from build123d import *

# Parameters (mm, degrees)
BOSS_EXTRUDE1_DEPTH = 8
HOLE1_D             = 3.2
HOLE1_CSINK_D       = 6
HOLE1_CSINK_ANGLE   = 90
FILLET1_R           = 5


with BuildPart() as part:
    # Sketch1 → Boss-Extrude1 (new body)
    with BuildSketch(Plane.XY):
        with BuildLine():
            Line((-13.754245124, 7.360756827), (-35.078110692, 7.360756827))
            Line((-35.078110692, 7.360756827), (-35.078110692, 1.360756827))
            Line((-35.078110692, 1.360756827), (-25.078110692, 1.360756827))
            Line((-25.078110692, 1.360756827), (-25.078110692, 4.360756827))
            Line((-25.078110692, 4.360756827), (-11.981080915, 4.360756827))
            ThreePointArc((-11.981080915, 4.360756827), (0, 12.75), (11.981080915, 4.360756827))
            Line((11.981080915, 4.360756827), (25.078110692, 4.360756827))
            Line((25.078110692, 4.360756827), (25.078110692, 1.360756827))
            Line((25.078110692, 1.360756827), (35.078110692, 1.360756827))
            Line((35.078110692, 1.360756827), (35.078110692, 7.360756827))
            Line((35.078110692, 7.360756827), (13.754245124, 7.360756827))
            ThreePointArc((13.754245124, 7.360756827), (0, 15.6), (-13.754245124, 7.360756827))
        make_face()
    extrude(amount=BOSS_EXTRUDE1_DEPTH)

    # Hole1 (through all)
    with Locations(Plane(origin=(-21.078110692, 7.360756827, 4), x_dir=(1, 0, 0), z_dir=(0, 1, 0))):
        with Locations((0, 0), (42.156221384, 0), (-10, 0), (52.156221384, 0)):
            CounterSinkHole(HOLE1_D / 2, HOLE1_CSINK_D / 2, counter_sink_angle=HOLE1_CSINK_ANGLE)

    # Fillet1
    fillet1_edges = [part.edges().sort_by_distance(p)[0] for p in [
        (-13.754245124, 7.360756827, 4),
        (13.754245124, 7.360756827, 4),
    ]]
    fillet(fillet1_edges, radius=FILLET1_R)


solid = part.part
Here's how the part is built. I have some questions about the finished solid (model axes, mm). A direction names the side the tool comes from. Coordinates: 2 decimals unless noted, no trailing zeros. Write each loop counter-clockwise with the first axis right and the second up, starting at its lowest first coordinate (ties: lowest second). Pieces come first, ordered by that corner, then holes. Notation, with made-up numbers: (85, 4) - (130, 4) arc R16 ccw to (130, 9) - close; hole circle Ø11 at (26, 15). An arc over 180 degrees is marked (long way). Use one line per item in the form item = value.
1) Thinking about a two-plate mould opening in Z: for faces 1 (the flat face through (0, 13, 0)), 2 (the cylindrical face through (-29.48, 3.63, 3.93)), 3 (the cylindrical face through (-22.6, 5.1, 3.5)), 4 (the flat face through (35.078, 4, 4)), which applies, released by +Z, released by -Z, zero draft, split by the parting line, or undercut?
Solved:
face_1 = released by -Z
face_2 = undercut
face_3 = undercut
face_4 = zero draft
2) On a 3-axis mill with a long thin cutter (end or side, diameter ignored), from which of +Z, -Z, +X, -X, +Y, -Y can I reach the whole of each face in a straight line? I mean faces 5 (the cylindrical face through (14.273, 7.874, 4.056)), 6 (the flat face through (18, 4.361, 4)), 7 (the flat face through (-26, 7.361, 4)). Say none if no direction works.
Solved:
face_5 = +Z, -Z, +X, +Y
face_6 = +Z, -Z, -Y
face_7 = +Z, -Z, -X, +Y
3) Suppose I cut it at D-D, the plane y = 14. Write out the boundary of the cut face in (x, z).
Solved:
outline = (-6.88, 0) - (6.88, 0) - (6.88, 8) - (-6.88, 8) - close
4) Suppose I cut it at B-B, the plane z = 4. Give the number of separate pieces and of enclosed holes in the cut face, plus the area to 3 significant figures.
Solved:
separate_pieces = 5
enclosed_holes = 0
area = 222 mm2
5) Suppose I cut it at A-A, the plane y = 8.5. Write out the boundary of the cut face in (x, z), plus the area to 3 significant figures.
Solved:
outline = (-13.3, 0) - (-9.5, 0) - (-9.5, 8) - (-13.3, 8) - close; (9.5, 0) - (13.3, 0) - (13.3, 8) - (9.5, 8) - close
area = 60.8 mm2
6) I'm going to push flat-ended pins straight in: P1, Ø4, axis at x = -30.5, z = 5, coming from the +Y side; P2, Ø4, axis at x = 4.5, z = 4.5, coming from the +Y side; P3, Ø4, axis at y = 12.5, z = 7, coming from the +X side; P4, Ø3, axis at x = -21.08, z = 4, coming from the +Y side. Where does each tip first touch, or does it pass through?
Solved:
P1 = 7.36
P2 = 15.4
P3 = 11.54
P4 = through
7) Suppose I cut it at C-C, the plane x = -2.5. Write out the boundary of the cut face in (y, z).
Solved:
outline = (12.5, 0) - (15.4, 0) - (15.4, 8) - (12.5, 8) - close
8) I need wall thicknesses on line 1 (X direction, y = 2.6, z = 4); line 2 (X direction, y = 5.65, z = 4); line 3 (Y direction, x = 26, z = 1.25). Which ranges of each line are inside material? Lowest first, please.
Solved:
line_1 = -35.08 to -32.68, -29.48 to -25.08, 25.08 to 29.48, 32.68 to 35.08
line_2 = -35.08 to -32.68, -29.48 to -22.68, -19.48 to -11.43, 11.43 to 19.48, 22.68 to 29.48, 32.68 to 35.08
line_3 = 1.36 to 7.36
